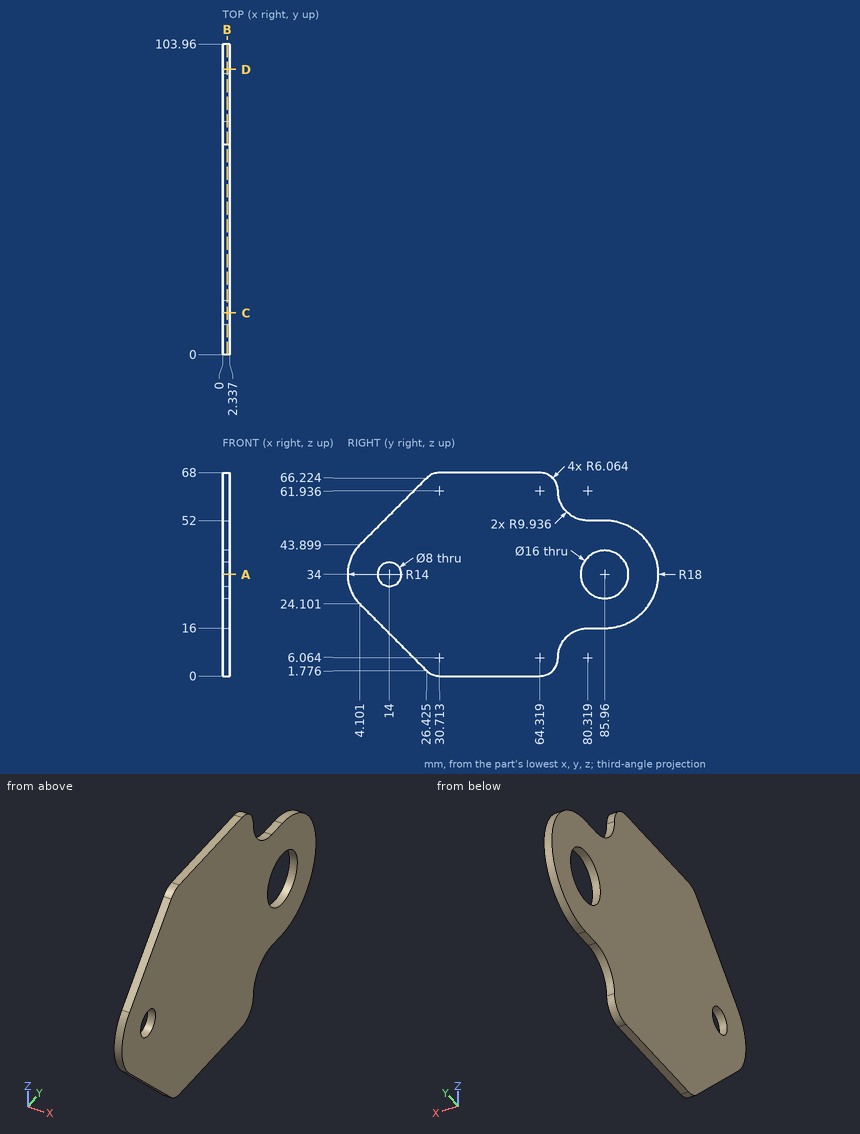
Geometry check sheet. Reference: drawing and pictorial views, mm from the part's lowest x, y, z. Give positions to 0.01 mm unless a question says otherwise; leave off trailing zeros. Loops run counter-clockwise (first coordinate to the right, second up) from the corner with the lowest first, then second, coordinate; pieces in that order, holes last. Notation, with made-up numbers: M -4,-3 L 6,-3 A16 ccw 6,18 Z; hole C 44.5,74 d5. An arc over 180 degrees is marked long. Use a Markdown table: item, result. Add a question column.
Q1. Sectioned sample at A-A, the plane z = 34. Record the cut outline in (x, y).
Q2. Sectioned sample at C-C, the plane y = 14. Record the cut outline in (x, z).
Q3. Go/stop test with flat-tipped pins: pin 1 (0.7 mm diameter, centred on x = 1.5, y = 84.5, fed in from -Z); pin 2 (1 mm diameter, centred on x = 0.5, z = 14.5, fed in from -Y). Record where each tip stops, or that it passes through.
Q4. Scan lines: line 1 along Y through (x, z) = (0.85, 34); line 2 along Z through (x, y) = (2.1, 80) (1 decimal); line 3 along Y through (x, z) = (0.75, 40). Record each from-to range of solid material in increasing order. Write a range as [from, to].
Q5. Sectioned sample at D-D, the plane y = 95.5. Record the cut outline in (x, z).
Q6. Sectioned sample at B-B, the plane x = 1.5. Record the cut outline in (y, z) (1 decimal), then the cut area to 3 significant figures.
Verdict:
| question | item | result |
|---|---|---|
| 1 | outline | M 0,0 L 2.34,0 L 2.34,10 L 0,10 Z; M 0,18 L 2.34,18 L 2.34,77.96 L 0,77.96 Z; M 0,93.96 L 2.34,93.96 L 2.34,103.96 L 0,103.96 Z |
| 2 | outline | M 0,14.2 L 2.34,14.2 L 2.34,30 L 0,30 Z; M 0,38 L 2.34,38 L 2.34,53.8 L 0,53.8 Z |
| 3 | pin 1 | z = 16 |
| 3 | pin 2 | y = 13.2 |
| 4 | line 1 | [0, 10], [18, 77.96], [93.96, 103.96] |
| 4 | line 2 | [16, 28.7], [39.3, 52] |
| 4 | line 3 | [1.35, 80.67], [91.25, 102.93] |
| 5 | outline | M 0,18.74 L 2.34,18.74 L 2.34,49.26 L 0,49.26 Z |
| 6 | outline | M 4.1,24.1 L 26.4,1.8 A6.1 ccw 30.7,0 L 64.3,0 A6.1 ccw 70.4,6.1 A9.9 cw 80.3,16 L 86,16 A18 ccw 86,52 L 80.3,52 A9.9 cw 70.4,61.9 A6.1 ccw 64.3,68 L 30.7,68 A6.1 ccw 26.4,66.2 L 4.1,43.9 A14 ccw Z; hole C 14,34 d8; hole C 86,34 d16 |
| 6 | area | 4,830 mm^2 |
